Source: CAD feature listing. Evaluate the final solid. Frame: model axes, mm. A direction names the side the tool comes from. Coordinates: 2 decimals unless noted, no trailing zeros. Order: outer loops, then holes, each group sorted by start corner. A loop starts at its lowest first (then second) coordinate and runs counter-clockwise, first axis right, second up.
```python
from build123d import *

# Parameters (mm, degrees)
SKETCH1_R            = 62.5
BOSS_EXTRUDE8_DEPTH  = 35
BOSS_EXTRUDE9_REACH  = 192.245
SKETCH2_W            = 15
SKETCH2_H            = 35
SKETCH10_W           = 35
SKETCH10_H           = 15
BOSS_EXTRUDE12_DEPTH = 40
SKETCH6_W            = 35
SKETCH6_H            = 15
BOSS_EXTRUDE10_DEPTH = 40
SKETCH11_W           = 20
SKETCH11_H           = 5
SKETCH11_W_2         = 25.5
SKETCH11_H_2         = 5.5
CUT_EXTRUDE1_DEPTH   = 20


with BuildPart() as part:
    # Sketch1 → Boss-Extrude8 (new body)
    with BuildSketch(Plane.XY):
        with BuildLine():
            Line((127.600917431, -117.745016448), (72.5, 0))
            ThreePointArc((72.5, 0), (0, 72.5), (-72.5, 0))
            Line((-72.5, 0), (-127.600917431, -117.745016448))
            Line((-127.600917431, -117.745016448), (-167.600917431, -117.745016448))
            Line((-167.600917431, -117.745016448), (-167.600917431, -137.745016448))
            Line((-167.600917431, -137.745016448), (167.600917431, -137.745016448))
            Line((167.600917431, -137.745016448), (167.600917431, -117.745016448))
            Line((167.600917431, -117.745016448), (127.600917431, -117.745016448))
        make_face()
        with BuildLine():
            ThreePointArc((-67.21559633, -27.171926873), (0, -72.5), (67.21559633, -27.171926873))
            Line((67.21559633, -27.171926873), (101.417450928, -100.25778678))
            Line((101.417450928, -100.25778678), (88.408256881, -117.745016448))
            Line((88.408256881, -117.745016448), (-88.408256881, -117.745016448))
            Line((-88.408256881, -117.745016448), (-101.417450928, -100.25778678))
            Line((-101.417450928, -100.25778678), (-67.21559633, -27.171926873))
        make_face(mode=Mode.SUBTRACT)
        Circle(SKETCH1_R, mode=Mode.SUBTRACT)
    extrude(amount=BOSS_EXTRUDE8_DEPTH)

    # Sketch2 → Boss-Extrude9 (add, up to next)
    with BuildSketch(Plane(origin=(0, -117.745016448, 0), x_dir=(1, 0, 0), z_dir=(0, 1, 0)), mode=Mode.PRIVATE) as boss_extrude9_sk1:
        with Locations((0.093911399, -17.5)):
            Rectangle(SKETCH2_W, SKETCH2_H)
    boss_extrude9_tool1 = extrude(boss_extrude9_sk1.sketch, amount=BOSS_EXTRUDE9_REACH, mode=Mode.PRIVATE) - part.part
    add(boss_extrude9_tool1.solids().sort_by_distance((0.093911, -117.745016, 17.5))[0])

    # Sketch10 → Boss-Extrude12 (add)
    with BuildSketch(Plane(origin=(-72.5, 0, 0), x_dir=(0, 0, -1), z_dir=(1, 0, 0))):
        with Locations((-17.5, -7.5)):
            Rectangle(SKETCH10_W, SKETCH10_H)
    extrude(amount=-BOSS_EXTRUDE12_DEPTH)

    # Sketch6 → Boss-Extrude10 (add)
    with BuildSketch(Plane(origin=(72.5, 0, 0), x_dir=(0, 0, -1), z_dir=(1, 0, 0))):
        with Locations((-17.5, -7.5)):
            Rectangle(SKETCH6_W, SKETCH6_H)
    extrude(amount=BOSS_EXTRUDE10_DEPTH)

    # Sketch11 → Cut-Extrude1 (cut)
    with BuildSketch(Plane.XY.offset(35)):
        with Locations((-92.5, -2.5)):
            Rectangle(SKETCH11_W, SKETCH11_H)
        with Locations((-92.5, -12.5)):
            Rectangle(SKETCH11_W, SKETCH11_H)
        with Locations((92.5, -2.5)):
            Rectangle(SKETCH11_W, SKETCH11_H)
        with Locations((92.5, -12.5)):
            Rectangle(SKETCH11_W, SKETCH11_H)
        with Locations((147.600917431, -120.495016448)):
            Rectangle(SKETCH11_W_2, SKETCH11_H_2)
        with Locations((147.600917431, -134.995016448)):
            Rectangle(SKETCH11_W_2, SKETCH11_H_2)
        with Locations((-147.600917431, -120.495016448)):
            Rectangle(SKETCH11_W_2, SKETCH11_H_2)
        with Locations((-147.600917431, -134.995016448)):
            Rectangle(SKETCH11_W_2, SKETCH11_H_2)
    extrude(amount=-CUT_EXTRUDE1_DEPTH, mode=Mode.SUBTRACT)


solid = part.part
```
1. Section query A-A on x = 0. Return loops of the section in (y, z), plus the area to 3 significant figures.
Findings:
outline: (-137.75, 0) - (-62.5, 0) - (-62.5, 35) - (-137.75, 35) - close; (62.5, 0) - (72.5, 0) - (72.5, 35) - (62.5, 35) - close
area: 2,980 mm2
2. Draft query along Y for faces 1 (the face through (103.9, -67.1, 17.3)), 2 (the face through (-1, -79, 0)), 3 (the face through (1.594, 72.482, 17.255)). Return one class per face: released by +Y, released by -Y, zero draft, split by the parting line, or undercut.
Findings:
face 1: undercut
face 2: zero draft
face 3: released by +Y
3. Ray query, line 1 (Y direction, x = 0, z = 21.5); line 2 (X direction, y = -121.5, z = 18); line 3 (Y direction, x = -56.5, z = 10). Return the intervals inside material, ascending.
Findings:
line 1: y = -137.75 to -62.5, 62.5 to 72.5
line 2: x = -167.6 to -160.35, -134.85 to 134.85, 160.35 to 167.6
line 3: y = -137.75 to -117.75, -45.43 to -26.72, 26.72 to 45.43
4. Pin query (flat end, axial travel): P1, Ø10.5, axis at x = 67.5, z = 12, coming from the +Y side; P2, Ø2.5, axis at y = -3.5, z = 23.5, coming from the +X side; P3, Ø17.5, axis at y = -90.5, z = 11, coming from the -X side. Return the tip coordinate at first contact, or that it passes through.
Findings:
P1: stops at y = 37.16
P2: stops at x = 112.5
P3: stops at x = -118.95
5. Section query B-B on z = 4. Return loops of the section in (x, y).
Findings:
outline: (-167.6, -137.75) - (167.6, -137.75) - (167.6, -117.75) - (127.6, -117.75) - (79.52, -15) - (112.5, -15) - (112.5, 0) - (72.5, 0) arc R72.5 ccw to (-72.5, 0) - (-112.5, 0) - (-112.5, -15) - (-79.52, -15) - (-127.6, -117.75) - (-167.6, -117.75) - close; hole (-101.42, -100.26) - (-88.41, -117.75) - (-7.41, -117.75) - (-7.41, -72.12) arc R72.5 cw to (-67.22, -27.17) - close; hole circle Ø125 at (0, 0); hole (7.59, -117.75) - (88.41, -117.75) - (101.42, -100.26) - (67.22, -27.17) arc R72.5 cw to (7.59, -72.1) - close
6. Section query C-C on x = -56. Return loops of the section in (y, z).
Findings:
outline: (-137.75, 0) - (-117.75, 0) - (-117.75, 35) - (-137.75, 35) - close; (-46.05, 0) - (-27.75, 0) - (-27.75, 35) - (-46.05, 35) - close; (27.75, 0) - (46.05, 0) - (46.05, 35) - (27.75, 35) - close
7. Access query for faces 4 (the face through (112.5, -7, 18)), 5 (the face through (7.594, -95, 18)), 6 (the face through (-148, -132.245, 25)), 7 (the face through (147, -123.245, 25)), 8 (the face through (-93, -10, 25)). Directions: +Z, -Z, +X, -X, +Y, -Y. A direction counts if a zero-diameter tool reaches every point of the face in a straight line with its end or side. Return the directions, or none.
Findings:
face 4: +Z, -Z, +X, +Y
face 5: +Z, -Z
face 6: +Z, -Y
face 7: +Z, +Y
face 8: +Z
8. Section query D-D on y = 15.5. Return loops of the section in (x, z), plus the area to 3 significant figures.
Findings:
outline: (-70.82, 0) - (-60.55, 0) - (-60.55, 35) - (-70.82, 35) - close; (60.55, 0) - (70.82, 0) - (70.82, 35) - (60.55, 35) - close
area: 719 mm2
